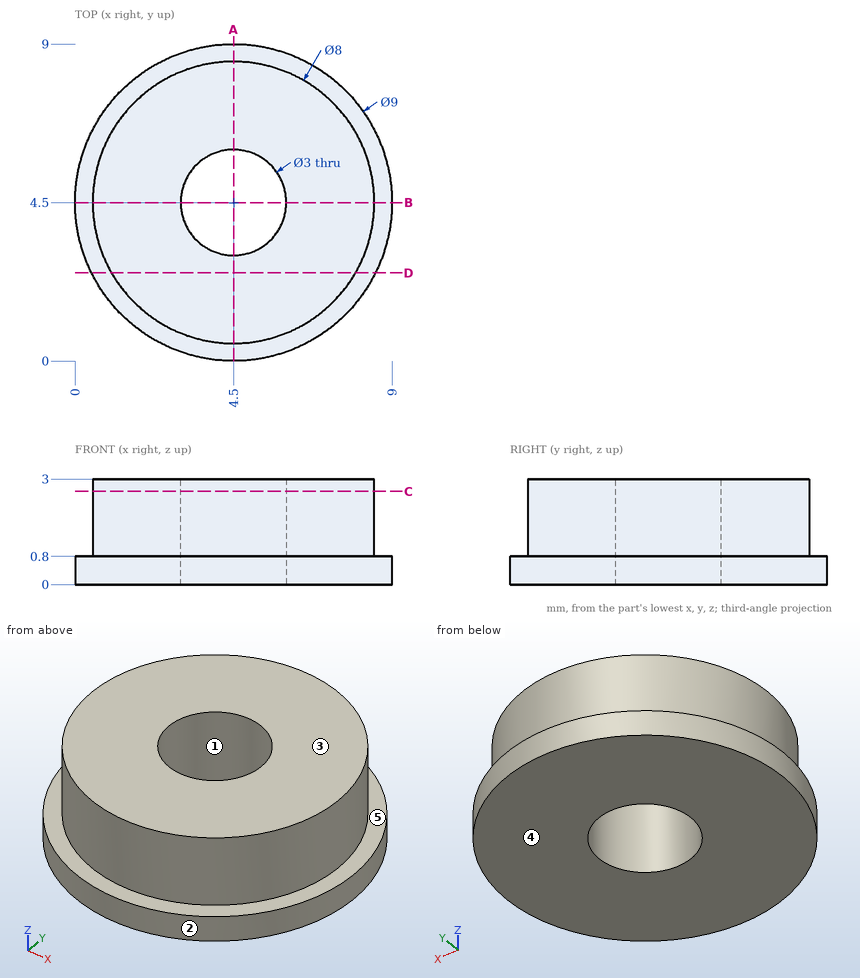
Study the drawing (mm; zero at the part's minimum x, y, z) and answer. A direction names the side the tool comes from. Coordinates: 2 decimals unless noted, no trailing zeros. Loops run counter-clockwise (first coordinate to the right, second up) from the corner with the lowest first, then second, coordinate; pieces in that order, holes last. Notation, with made-up numbers: M 59.25,45 L 113.25,45 A19 cw 113.25,76 Z; hole C 37,-39.5 d5. An arc over 180 degrees is marked long. Answer as a JSON object with one key per item and string values. Group by question number.
Item 1: Consider L1, parallel to Y at x = 4.5, z = 1; L2, parallel to Z at x = 1.25, y = 1.5; L3, parallel to Y at x = 3.5, z = 2.95. Determine where each line is inside the solid, lowest interval first.
Item 2: Section C-C (z = 2.65) is taken. Write down the section's boundary in (x, y), and give its area (3 significant figures).
Item 3: Which of the six approach directions +Z, -Z, +X, -X, +Y, -Y give full straight-line access (tool end or side, diameter ignored) to the marked faces 4 and 5?
Item 4: Each of these flat-tipped pins is pushed along its axis until it touches: P1, Ø1, axis at y = 2.5, z = 0.5, coming from the +X side; P2, Ø2.5, axis at x = 4.5, y = 4.5, coming from the -Z side. Where does it stop, or does it pass through?
Item 5: Section A-A (x = 4.5) is taken. Write down the section's boundary in (y, z), and give its area (3 significant figures).
Item 6: Determine the mould class of the marked faces 1, 2 and 3 for opening direction X: +X half, -X half, draft (parallel to the pull), parting line (faces both ways), or undercut.
Item 7: Section D-D (y = 2.5) is taken. Write down the section's boundary in (x, z), and give its area (3 significant figures).
Solved:
{
 "1": {"L1": "y = 0.5 to 3, 6 to 8.5", "L2": "z = 0 to 0.8", "L3": "y = 0.63 to 3.38, 5.62 to 8.37"},
 "2": {"outline": "C 4.5,4.5 d8; hole C 4.5,4.5 d3", "area": "43.2 mm2"},
 "3": {"face 4": "-Z, +X, -X, +Y, -Y", "face 5": "+Z"},
 "4": {"P1": "stops at x = 8.74", "P2": "passes through"},
 "5": {"outline": "M 0,0 L 3,0 L 3,3 L 0.5,3 L 0.5,0.8 L 0,0.8 Z; M 6,0 L 9,0 L 9,0.8 L 8.5,0.8 L 8.5,3 L 6,3 Z", "area": "15.8 mm2"},
 "6": {"face 1": "undercut", "face 2": "parting line", "face 3": "draft"},
 "7": {"outline": "M 0.47,0 L 8.53,0 L 8.53,0.8 L 7.96,0.8 L 7.96,3 L 1.04,3 L 1.04,0.8 L 0.47,0.8 Z", "area": "21.7 mm2"}
}
